from build123d import *

# Parameters (mm, degrees)
SKETCH_1_R          = 13.5
SKETCH_1_R_2        = 10
EXTRUDE_1_DEPTH     = 4
SKETCH_2_R          = 12.72
SKETCH_2_R_2        = 11.2
CUT_EXTRUDE_1_DEPTH = 0.5
SKETCH_3_R          = 12.72
SKETCH_3_R_2        = 11.2
CUT_EXTRUDE_2_DEPTH = 0.5


with BuildPart() as part:
    # 草圖1 → 填料-伸長1 (new body)
    with BuildSketch(Plane.XY):
        Circle(SKETCH_1_R)
        Circle(SKETCH_1_R_2, mode=Mode.SUBTRACT)
    extrude(amount=EXTRUDE_1_DEPTH)

    # 草圖2 → 除料-伸長1 (cut)
    with BuildSketch(Plane.XY.offset(4)):
        Circle(SKETCH_2_R)
        Circle(SKETCH_2_R_2, mode=Mode.SUBTRACT)
    extrude(amount=-CUT_EXTRUDE_1_DEPTH, mode=Mode.SUBTRACT)

    # 草圖3 → 除料-伸長2 (cut)
    with BuildSketch(Plane(origin=(0, 0, 0), x_dir=(-1, 0, 0), z_dir=(0, 0, -1))):
        Circle(SKETCH_3_R)
        Circle(SKETCH_3_R_2, mode=Mode.SUBTRACT)
    extrude(amount=-CUT_EXTRUDE_2_DEPTH, mode=Mode.SUBTRACT)


solid = part.part
Can you work these out from the model? Positions are in its coordinate system, mm. A direction names the side the tool comes from. Give positions to 0.01 mm unless a question says otherwise; leave off trailing zeros. Order: outer loops, then holes, each group sorted by start corner. A loop starts at its lowest first (then second) coordinate and runs counter-clockwise, first axis right, second up. Notation, with made-up numbers: M -32,29.5 L -12,29.5 A16 ccw -12,55.5 Z; hole C 24.5,2.5 d8. An arc over 180 degrees is marked long. Use a Markdown table: item, result. Add a question column.
Item 1: Suppose I cut it at D-D (x = 11.75). List the corners of the cut face in (y, z) for me, then the cut area to 3 significant figures.
Item 2: We'd pull the mould along X, two halves only. Please class faces 4 (the flat face through (-8, 7, 0)), 5 (the cylindrical face through (2.757, -12.418, 0.246)), 6 (the flat face through (-7, -9, 0.5)), 7 (the cylindrical face through (-2.93, -13.18, 1.97)): +X half, -X half, draft (parallel to the pull), parting line (faces both ways), or undercut.
Item 3: For faces 1 (the flat face through (-10.1, 8.1, 0)), 2 (the cylindrical face through (-11.19, 0.49, 3.75)), 3 (the cylindrical face through (11.19, 0.49, 0.25)), which set-ups out of +Z, -Z, +X, -X, +Y, -Y let a thin tool reach every point of the face, with its end or its side?
Item 4: If I drill on L1, parallel to Y at x = 0, z = 0.4; L2, parallel to X at y = 5.5, z = 0.35; L3, parallel to X at y = 0.5, z = 0.2, over which ranges is the centre line in solid material (lowest first)? Write a range as [from, to].
Item 5: Will these pins go through, and if not, where does the flat tip stop? pin 1 (2 mm diameter, centred on x = 4.5, z = 3, fed in from +Y); pin 2 (1 mm diameter, centred on x = 6, z = 2, fed in from +Y); pin 3 (15.5 mm diameter, centred on x = 0, y = 0, fed in from -Z).
Item 6: Suppose I cut it at C-C (z = 1.2). List the corners of the cut face in (x, y) for me.
Item 7: Suppose I cut it at A-A (x = 0). List the corners of the cut face in (y, z) for me, then the cut area to 3 significant figures.
Answer sheet:
| question | item | result |
|---|---|---|
| 1 | outline | M -6.65,0 L -4.87,0 L -4.87,0.5 L 4.87,0.5 L 4.87,0 L 6.65,0 L 6.65,4 L 4.87,4 L 4.87,3.5 L -4.87,3.5 L -4.87,4 L -6.65,4 Z |
| 1 | area | 43.4 mm² |
| 2 | face 4 | draft |
| 2 | face 5 | undercut |
| 2 | face 6 | undercut |
| 2 | face 7 | parting line |
| 3 | face 1 | -Z, +X, -X, +Y, -Y |
| 3 | face 2 | +Z |
| 3 | face 3 | -Z |
| 4 | L1 | y = [-13.5, -12.72], [-11.2, -10], [10, 11.2], [12.72, 13.5] |
| 4 | L2 | x = [-12.33, -11.47], [-9.76, -8.35], [8.35, 9.76], [11.47, 12.33] |
| 4 | L3 | x = [-13.49, -12.71], [-11.19, -9.99], [9.99, 11.19], [12.71, 13.49] |
| 5 | pin 1 | stops at y = 13.04 |
| 5 | pin 2 | stops at y = 12.33 |
| 5 | pin 3 | passes through |
| 6 | outline | C 0,0 d27; hole C 0,0 d20 |
| 7 | outline | M -13.5,0 L -12.72,0 L -12.72,0.5 L -11.2,0.5 L -11.2,0 L -10,0 L -10,4 L -11.2,4 L -11.2,3.5 L -12.72,3.5 L -12.72,4 L -13.5,4 Z; M 10,0 L 11.2,0 L 11.2,0.5 L 12.72,0.5 L 12.72,0 L 13.5,0 L 13.5,4 L 12.72,4 L 12.72,3.5 L 11.2,3.5 L 11.2,4 L 10,4 Z |
| 7 | area | 25.0 mm² |
